Check sheet for the modelled part. Datum: model origin and axes. Units: mm. Face numbers are marked on the shaded views. Round coordinates to 2 decimals unless told otherwise and drop trailing zeros. Loops run counter-clockwise (first coordinate to the right, second up) from the corner with the lowest first, then second, coordinate; pieces in that order, holes last. Notation, with made-up numbers: (-8.75, 37) -> (25.25, 37) arc R22 cw to (25.25, 70) -> close; hole circle Ø7 at (72.25, 44.25). An arc over 180 degrees is marked (long way). Return JSON: item names as keys, results as strings.
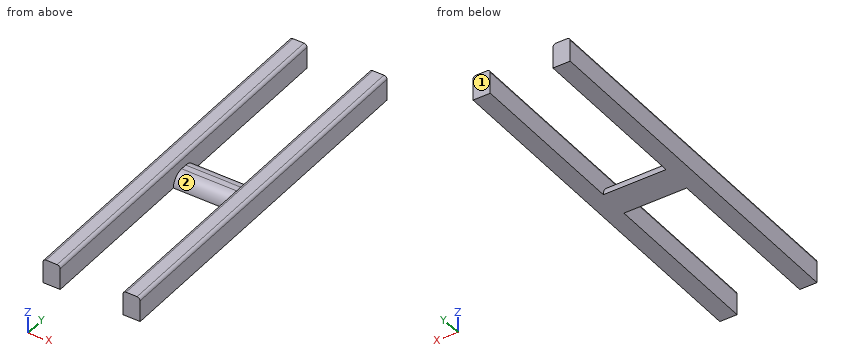
from build123d import *

# Parameters (mm, degrees)
F1_DEPTH = 76.2
F0_W     = 25.8755748077
F0_H     = 5.08
F2_DEPTH = 6.35
F3_R     = 1.27
F4_R     = 5.07999


# Not quite as in the source:
# - two fillets or chamfers of one size are made in one step
# - a fillet or chamfer is up to 0.001 mm smaller than in the source, because OpenCascade refuses the exact size


with BuildPart() as f1:
    # F0 (on Front) → F1 (new body, symmetric)
    with BuildSketch(Plane.XZ):
        Polygon((-38.5863832052, 10.16), (-45.6983832052, 10.16), (-45.6983832052, 0), (-38.5863832052, 0), (-38.5863832052, 5.08), align=None)
    extrude(amount=F1_DEPTH, both=True)



with BuildPart() as f1b:
    # F0 (on Front) → F1, piece 2 (new body, symmetric)
    with BuildSketch(Plane.XZ):
        Polygon((-12.7108083974, 10.16), (-12.7108083974, 5.08), (-12.7108083974, 0), (-5.5988083974, 0), (-5.5988083974, 10.16), align=None)
    extrude(amount=F1_DEPTH, both=True)


with BuildPart() as f1_1:
    add(f1.part)

    add(f1b.part)  # F2 merges F1b
    # F0 (on Front) → F2 (join, symmetric)
    with BuildSketch(Plane.XZ):
        Polygon((-38.5863832052, 10.16), (-45.6983832052, 10.16), (-45.6983832052, 0), (-38.5863832052, 0), (-38.5863832052, 5.08), align=None)
        with Locations((-25.6485958013, 2.54)):
            Rectangle(F0_W, F0_H)
        Polygon((-12.7108083974, 10.16), (-12.7108083974, 5.08), (-12.7108083974, 0), (-5.5988083974, 0), (-5.5988083974, 10.16), align=None)
    extrude(amount=F2_DEPTH, both=True)

    # F3
    f3_edges = [f1_1.edges().sort_by_distance(p)[0] for p in [
        (-45.698383, 0, 10.16),
        (-38.586383, 0, 10.16),
        (-12.710808, 0, 10.16),
        (-5.598808, 0, 10.16),
    ]]
    fillet(f3_edges, radius=F3_R)

    # F4 (radius 5.08 in the source; OpenCascade refuses exactly that, so slightly less here)
    f4_edges = [f1_1.edges().sort_by_distance(p)[0] for p in [
        (-25.648596, 6.35, 5.08),
        (-25.648596, -6.35, 5.08),
    ]]
    fillet(f4_edges, radius=F4_R)


solid = f1_1.part
Q1. Section check B-B (z = 7.25). Record the boundary of the cut face in (x, y), then the cut area to 3 significant figures.
Results list:
{"outline": "(-45.7, -76.2) -> (-38.59, -76.2) -> (-38.59, 76.2) -> (-45.7, 76.2) -> close; (-12.71, -76.2) -> (-5.6, -76.2) -> (-5.6, 76.2) -> (-12.71, 76.2) -> close", "area": "2,170 mm^2"}
Q2. Go/stop test with flat-tipped pins: pin 1 (4 mm diameter, centred on x = -19, z = 8.5, fed in from +Y); pin 2 (3 mm diameter, centred on x = -29.5, y = -0.5, fed in from +Z); pin 3 (4 mm diameter, centred on x = -18, z = 2, fed in from -Y). Record where each tip stops, or that it passes through.
Results list:
{"pin 1": "through", "pin 2": "z = 5.08", "pin 3": "y = -6.35"}
Q3. Draft check along X on the marked faces 1 and 2. Enter one of: released by +X, released by -X, zero draft, split by the parting line, or undercut.
Results list:
{"face 1": "zero draft", "face 2": "undercut"}
Q4. Material ranges on line 1 (X direction, y = -0.5, z = 7.75); line 2 (X direction, y = 46.5, z = 9.25); line 3 (Z direction, x = -11.5, y = -46), recorded low to high.
Results list:
{"line 1": "-45.7 to -38.59, -12.71 to -5.6", "line 2": "-45.65 to -38.64, -12.66 to -5.65", "line 3": "0 to 10.16"}
Q5. Section check A-A (y = 49). Record the boundary of the cut face in (x, z).
Results list:
{"outline": "(-45.7, 0) -> (-38.59, 0) -> (-38.59, 8.89) arc R1.27 ccw to (-39.86, 10.16) -> (-44.43, 10.16) arc R1.27 ccw to (-45.7, 8.89) -> close; (-12.71, 0) -> (-5.6, 0) -> (-5.6, 8.89) arc R1.27 ccw to (-6.87, 10.16) -> (-11.44, 10.16) arc R1.27 ccw to (-12.71, 8.89) -> close"}
